Autodesk Inventor part; units mm, degrees
ref_plane "YZ Plane" through (0, 0, 0) normal (1, 0, 0) x (0, 1, 0)
ref_plane "XZ Plane" through (0, 0, 0) normal (0, 1, 0) x (-1, 0, 0)
ref_plane "XY Plane" through (0, 0, 0) normal (0, 0, 1) x (1, 0, 0)
sketch "Skizze1" plane through (0, 0, 0) normal (0, 0, 1) x (1, 0, 0)
  line L0 (0, 0) -> (30, 0)
  line L1 (30, 0) -> (30, 40)
  line L2 (30, 40) -> (0, 40)
  line L3 (0, 40) -> (0, 0)
  dimension "d0" = 30
  dimension "d1" = 40
extrude "Extrusion1" add sketch "Skizze1" along normal blind 10
sketch "Skizze2" plane through (0, 0, 10) normal (0, 0, 1) x (1, 0, 0)
  line L0 (5, 27.5) -> (25, 27.5) construction
  line L1 (25, 27.5) -> (25, 12.5) construction
  line L2 (25, 12.5) -> (5, 12.5) construction
  line L3 (5, 12.5) -> (5, 27.5) construction
  line L4 (30, 40) -> (0, 40) construction
  line L5 (15, 27.5) -> (15, 40) construction
  line L6 (15, 12.5) -> (15, 0) construction
  line L7 (0, 0) -> (30, 0)
  dimension "d5" = 15
  dimension "d8" = 20
hole "Bohrung1" at (5, 27.5, 10) at (25, 27.5, 10) at (25, 12.5, 10) at (5, 12.5, 10) direction (0, 0, -1) diameter 3.4 end through all counterbore diameter 6.5 counterbore depth 3.4
sketch "Skizze3" plane through (0, 0, 0) normal (0, 0, -1) x (-1, 0, 0)
  line L0 (-18.5, 40) -> (-11.5, 40)
  line L1 (-11.5, 40) -> (-11.5, 15)
  line L2 (-11.5, 15) -> (-18.5, 15)
  line L3 (-18.5, 15) -> (-18.5, 40)
  line L4 (-30, 40) -> (0, 40)
  point P0 (0, 0)
  point P1 (-15, 40)
  dimension "d19" = 7
  dimension "d20" = 25
extrude "Extrusion2" cut sketch "Skizze3" against normal blind 0.5
fillet "Rundung3" radius 0.5 4 edges at (18.5, 40, 0.25) (11.5, 40, 0.25) (18.5, 15, 0.25) (11.5, 15, 0.25)
fillet "Rundung1" radius 5 4 edges at (0, 40, 5) (30, 40, 5) (0, 0, 5) (30, 0, 5)
fillet "Rundung2" radius 0.5 17 edges at (1.4645, 1.4645, 0) (15, 0, 0) (28.5355, 1.4645, 0) (30, 20, 0) (28.5355, 38.5355, 0) (8, 40, 0) (22, 40, 0) (1.4645, 38.5355, 0) (0, 20, 0) (1.4645, 38.5355, 10) (0, 20, 10) (1.4645, 1.4645, 10) (15, 0, 10) (28.5355, 1.4645, 10) (30, 20, 10) (28.5355, 38.5355, 10) (15, 40, 10)
sketch "Skizze4" plane through (0, 0, 10) normal (0, 0, 1) x (1, 0, 0)
  line L0 (19, 40) -> (11, 40) construction
  line L1 (15, 40) -> (15, 32.5) construction
  line L2 (15, 32.5) -> (15, 7.5) construction
  line L3 (15, 7.5) -> (15, 0) construction
  line L4 (25, 0) -> (5, 0) construction
  point P0 (0, 0)
  dimension "d24" = 25
hole "Bohrung2" at (15, 32.5, 10) at (15, 7.5, 10) direction (0, 0, -1) diameter 4 end through all
properties part number "AdapterLinearGuideShort"
The model under review builds one solid part; all positions refer to its coordinate system, in mm. A direction names the side the tool comes from. Round coordinates to 2 decimals unless told otherwise and drop trailing zeros. Order: outer loops, then holes, each group sorted by start corner. A loop starts at its lowest first (then second) coordinate and runs counter-clockwise, first axis right, second up.
(1) For P1, Ø2, axis at x = 25, y = 26.5, coming from the +Z side; P2, Ø6.5, axis at x = 15, y = 32.5, coming from the -Z side, all flat-tipped, find the tip position at first contact; note any pin that passes through.
Working result:
P1: stops at z = 6.6
P2: stops at z = 0.5
(2) Tool access review of faces 1 (the face through (14, 28, 0.5)), 2 (the face through (15, 0, 5)), 3 (the face through (26.245, 24.498, 8.276)): name each direction out of +Z, -Z, +X, -X, +Y, -Y from which nothing blocks a thin tool from reaching the whole face with its end or side.
Working result:
face 1: -Z, +Y
face 2: +Z, -Z, +X, -X, -Y
face 3: +Z
(3) Take a section at B-B, the plane y = 12.5. State the section outline as (x, z) points.
Working result:
outline: (0, 0.5) arc R0.5 ccw to (0.5, 0) - (3.3, 0) - (3.3, 6.6) - (1.75, 6.6) - (1.75, 10) - (0.5, 10) arc R0.5 ccw to (0, 9.5) - close; (6.7, 0) - (23.3, 0) - (23.3, 6.6) - (21.75, 6.6) - (21.75, 10) - (8.25, 10) - (8.25, 6.6) - (6.7, 6.6) - close; (26.7, 0) - (29.5, 0) arc R0.5 ccw to (30, 0.5) - (30, 9.5) arc R0.5 ccw to (29.5, 10) - (28.25, 10) - (28.25, 6.6) - (26.7, 6.6) - close
(4) Wall thickness on L1, parallel to X at y = 27.5, z = 8.1; L2, parallel to Y at x = 15, z = 7; L3, parallel to Y at x = 25, z = 1.75: over which ranges is each line inside the solid? List them lowest first.
Working result:
L1: x = 0 to 1.75, 8.25 to 21.75, 28.25 to 30
L2: y = 0 to 5.5, 9.5 to 30.5, 34.5 to 40
L3: y = 0 to 10.8, 14.2 to 25.8, 29.2 to 40
(5) Take a section at C-C, the plane x = 15. Count the separate pieces of the cut face and the enclosed holes in it, plus the area to 3 significant figures.
Working result:
separate pieces: 3
enclosed holes: 0
area: 309 mm2
(6) Mouldability with a two-part tool opening along Y and no side actions: class faces 4 (the face through (15, 20, 10)), 5 (the face through (13.648, 8.974, 4.93)), 6 (the face through (29, 38, 5)) as released by +Y, released by -Y, zero draft, split by the parting line, or undercut.
Working result:
face 4: zero draft
face 5: undercut
face 6: released by +Y
(7) Take a section at D-D, the plane z = 2.25. State the section outline as (x, y) points, plus the area to 3 significant figures.
Working result:
outline: (0, 5) arc R5 ccw to (5, 0) - (25, 0) arc R5 ccw to (30, 5) - (30, 35) arc R5 ccw to (25, 40) - (5, 40) arc R5 ccw to (0, 35) - close; hole circle Ø3.4 at (5, 12.5); hole circle Ø3.4 at (5, 27.5); hole circle Ø4 at (15, 7.5); hole circle Ø4 at (15, 32.5); hole circle Ø3.4 at (25, 12.5); hole circle Ø3.4 at (25, 27.5)
area: 1,120 mm2
